CAD build for the part. Positions are in the model's coordinates, mm. A direction names the side the tool comes from. Give positions to 0.01 mm unless a question says otherwise; leave off trailing zeros. Loops run counter-clockwise (first coordinate to the right, second up) from the corner with the lowest first, then second, coordinate; pieces in that order, holes last.
```python
from build123d import *

# Parameters (mm, degrees)
EXTRUDE_1_DEPTH = 10
CHAMFER_1_SIZE  = 5


with BuildPart() as part:
    # 草图1 → 凸台-拉伸1 (new body)
    with BuildSketch(Plane.ZY):
        with BuildLine():
            Line((6.100444343, 13.976661934), (-21, 25.805291199))
            Line((-21, 25.805291199), (-14.999562941, 39.552827528))
            Line((-14.999562941, 39.552827528), (12.100881401, 27.724198263))
            ThreePointArc((12.100881401, 27.724198263), (30.25, 0), (12.100881401, -27.724198263))
            Line((12.100881401, -27.724198263), (-14.999562941, -39.552827528))
            Line((-14.999562941, -39.552827528), (-21, -25.805291199))
            Line((-21, -25.805291199), (6.100444343, -13.976661934))
            ThreePointArc((6.100444343, -13.976661934), (15.25, 0), (6.100444343, 13.976661934))
        make_face()
    extrude(amount=EXTRUDE_1_DEPTH)

    # 倒角1
    chamfer_1_edges = [part.edges().sort_by_distance(p)[0] for p in [
        (0, -33.638512895, -1.44934077),
        (0, 33.638512895, -1.44934077),
        (0, 0, 30.25),
    ]]
    chamfer(chamfer_1_edges, length=CHAMFER_1_SIZE)


solid = part.part
```
1. Probe line 1 along Y through (x, z) = (-7.75, -17); line 2 along Y through (x, z) = (-9.25, -18); line 3 along Z through (x, y) = (-8.25, 12). List the from-to ranges inside material, lowest first.
Responses:
line 1: y = -34.97 to -24.06, 24.06 to 34.97
line 2: y = -32.68 to -24.5, 24.5 to 32.68
line 3: z = 9.41 to 27.77
2. Tool access for faces 4 (the face through (-4.93, 19.81, -7.26)), 5 (the face through (-4.93, 32.583, -18.042)): list every direction of +Z, -Z, +X, -X, +Y, -Y with a clear straight run to the whole face (end or side of a thin tool).
Responses:
face 4: -Z, +X, -X
face 5: -Z, +X, -X, +Y
3. Saw through at D-D, the plane x = -1. List the corners of the cut face in (y, z).
Responses:
outline: (-35.89, -16.6) - (-25.81, -21) - (-13.98, 6.1) arc R15.25 cw to (13.98, 6.1) - (25.81, -21) - (35.89, -16.6) - (24.06, 10.5) arc R26.25 ccw to (-24.06, 10.5) - close
4. Saw through at B-B, the plane x = -9. List the corners of the cut face in (y, z).
Responses:
outline: (-39.55, -15) - (-25.81, -21) - (-13.98, 6.1) arc R15.25 cw to (13.98, 6.1) - (25.81, -21) - (39.55, -15) - (27.72, 12.1) arc R30.25 ccw to (-27.72, 12.1) - close
5. Drop flat-ended pins along their axis: pin 1 (5 mm diameter, centred on x = -1, z = 10.5, fed in from -Y); pin 2 (1.5 mm diameter, centred on x = -7.5, z = 12.5, fed in from +Y); pin 3 (3 mm diameter, centred on x = -2.5, y = -25, fed in from +Z). Give the stop position or say it passes through.
Responses:
pin 1: stops at y = -27
pin 2: stops at y = 27.88
pin 3: stops at z = 16.04
6. Pull direction Y, two halves, no side cores. Call faces 1 (the face through (-0.243, 0.414, 25.489)), 2 (the face through (-4.93, -0.247, 15.248)), 3 (the face through (-10, 1, 16)): released by +Y, released by -Y, zero draft, split by the parting line, or undercut.
Responses:
face 1: split by the parting line
face 2: undercut
face 3: zero draft
7. Saw through at C-C, the plane y = 29.5. List the corners of the cut face in (x, z), and give its area (3 significant figures).
Responses:
outline: (-10, -19.39) - (0, -19.39) - (0, -4.47) - (-5, 8.03) - (-10, 8.03) - close
area: 243 mm2
8. Saw through at A-A, the plane z = 7.5. List the corners of the cut face in (x, y), and give its area (3 significant figures).
Responses:
outline: (-10, -29.73) - (-5, -29.73) - (0, -24.28) - (0, -13.28) - (-10, -13.28) - close; (-10, 13.28) - (0, 13.28) - (0, 24.28) - (-5, 29.73) - (-10, 29.73) - close
area: 302 mm2
